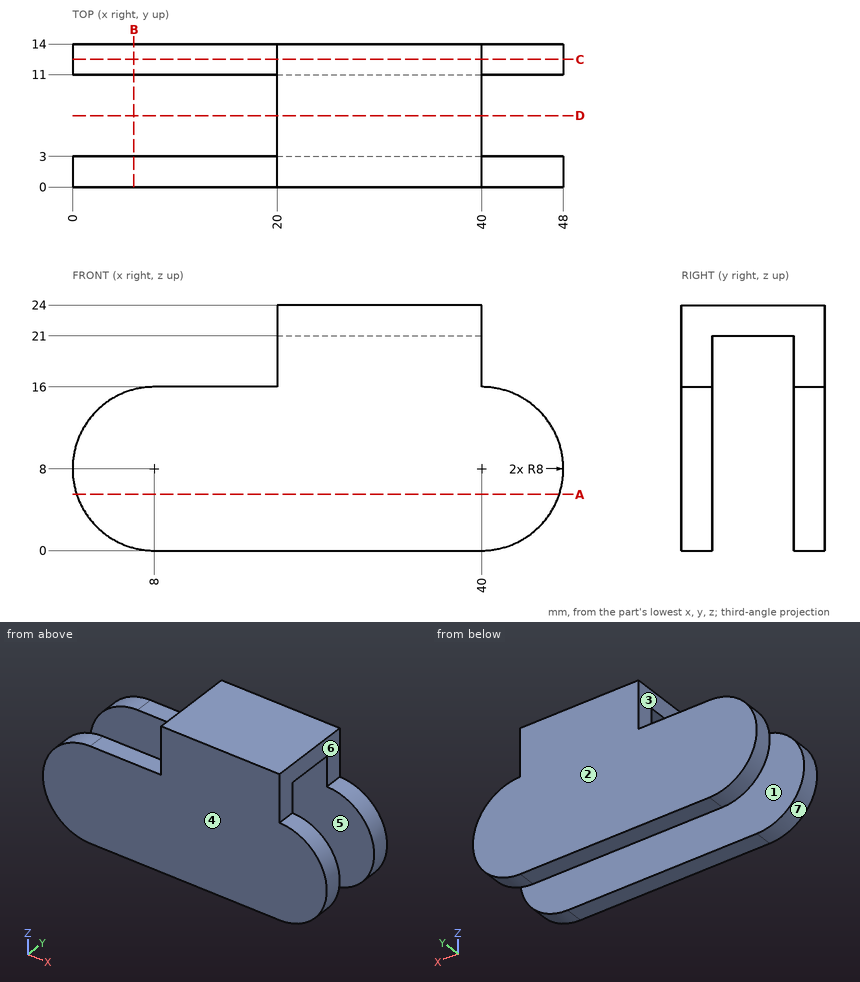
Check sheet for the drawn part. Datum: minimum x, y, z corner. Units: mm. A direction names the side the tool comes from. Round coordinates to 2 decimals unless told otherwise and drop trailing zeros. Order: outer loops, then holes, each group sorted by start corner. A loop starts at its lowest first (then second) coordinate and runs counter-clockwise, first axis right, second up.
1. Section check D-D on y = 7. Record the cut outline in (x, z), then the cut area to 3 significant figures.
Final values:
outline: (20, 21) - (40, 21) - (40, 24) - (20, 24) - close
area: 60.0 mm2
2. Release check for a two-part mould opening along Y. For the marked faces 1, 2, 3 and 4 record: +Y half, -Y half, draft (parallel to the pull), parting line (faces both ways), or undercut.
Final values:
face 1: undercut
face 2: +Y half
face 3: draft
face 4: -Y half
3. Go/stop test with flat-tipped pins: P1, Ø0.9, axis at x = 11.5, y = 1.5, coming from the +Z side; P2, Ø4, axis at y = 8.5, z = 19.5, coming from the +X side; P3, Ø2.5, axis at y = 7, z = 19.5, coming from the -X side. Record where each tip stops, or that it passes through.
Final values:
P1: stops at z = 16
P2: stops at x = 40
P3: passes through
4. Access from +Z, -Z, +X, -X, +Y, -Y to the whole of each face (thin tool, end or side, straight path). Record for the marked faces 5, 6 and 7.
Final values:
face 5: -Z, +X, -X
face 6: +Z, +X, +Y, -Y
face 7: -X, +Y, -Y
5. Section check A-A on z = 5.5. Record the cut outline in (x, y), then the cut area to 3 significant figures.
Final values:
outline: (0.4, 0) - (47.6, 0) - (47.6, 3) - (0.4, 3) - close; (0.4, 11) - (47.6, 11) - (47.6, 14) - (0.4, 14) - close
area: 283 mm2
6. Section check B-B on x = 6. Record the cut outline in (y, z).
Final values:
outline: (0, 0.25) - (3, 0.25) - (3, 15.75) - (0, 15.75) - close; (11, 0.25) - (14, 0.25) - (14, 15.75) - (11, 15.75) - close
7. Section check C-C on y = 12.5. Record the cut outline in (x, z).
Final values:
outline: (8, 0) - (40, 0) arc R8 ccw to (40, 16) - (40, 24) - (20, 24) - (20, 16) - (8, 16) arc R8 ccw to start
8. Thickness scan on L1, parallel to Y at x = 39.5, z = 18.75; L2, parallel to Z at x = 38, y = 4.25; L3, parallel to X at y = 1.25, z = 7.75. Record the ranges inside material, lowest first.
Final values:
L1: y = 0 to 3, 11 to 14
L2: z = 21 to 24
L3: x = 0 to 48
